CAD build for the part. Positions are in the model's coordinates, mm. Coordinates: 2 decimals unless noted, no trailing zeros. Order: outer loops, then holes, each group sorted by start corner. A loop starts at its lowest first (then second) coordinate and runs counter-clockwise, first axis right, second up. Notation, with made-up numbers: M 52.5,12 L 76.5,12 A16 cw 76.5,25 Z; hole C 50,-36.75 d10. An arc over 180 degrees is marked long. One line per item, written item: value.
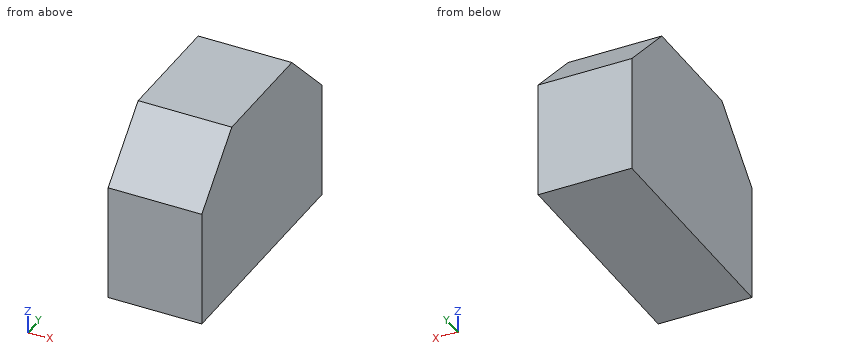
from build123d import *

# Parameters (mm, degrees)
F0_W     = 80
F0_H     = 200
F1_DEPTH = 150
F2_SIZE  = 50


with BuildPart() as f1:
    # F0 (on Top) → F1 (new body)
    with BuildSketch(Plane.XY):
        with Locations((40, -100)):
            Rectangle(F0_W, F0_H)
    extrude(amount=F1_DEPTH)

    # F2
    f2_edges = [f1.edges().sort_by_distance(p)[0] for p in [
        (40, 0, 150),
        (40, -200, 150),
    ]]
    chamfer(f2_edges, length=F2_SIZE)


solid = f1.part
Q1. Slice it at C-C (z = 126.5). List the corners of the cut face in (x, y).
Recorded:
outline: M 0,-173.5 L 80,-173.5 L 80,-26.5 L 0,-26.5 Z
Q2. Slice it at A-A (x = 24). List the corners of the cut face in (y, z), plus the area to 3 significant figures.
Recorded:
outline: M -200,0 L 0,0 L 0,100 L -50,150 L -150,150 L -200,100 Z
area: 27,500 mm^2
Q3. Pin check, flat tip, straight feed: pin 1 Ø1 at (y, z) = (-60, 97.5) entering from -X. Stop position of the tip, or through.
Recorded:
pin 1: stops at x = 0
Q4. Slice it at B-B (y = -153.5). List the corners of the cut face in (x, z).
Recorded:
outline: M 0,0 L 80,0 L 80,146.5 L 0,146.5 Z
Q5. Drill centre lines: line 1 along Y through (x, z) = (9, 124); line 2 along Z through (x, y) = (32, -176.5); line 3 along Y through (x, z) = (61.5, 104). Where is each one in solid material? Low to high.
Recorded:
line 1: y = -176 to -24
line 2: z = 0 to 123.5
line 3: y = -196 to -4
